from build123d import *

# Parameters (mm, degrees)
SKETCH001_W                   = 44
SKETCH001_H                   = 15
POCKET_DEPTH                  = 325.585135
PAD_DEPTH                     = 22.25
SKETCH003_W                   = 28
SKETCH003_H                   = 15
POCKET001_DEPTH               = 325.585135
SKETCH004_R                   = 1.5
POCKET002_DEPTH               = 45
SKETCH004_MIRRORED014_2_R     = 1.5
POCKET002_MIRRORED014_2_DEPTH = 45
SKETCH006_R                   = 1.2
POCKET004_DEPTH               = 325.585135
SKETCH006_MIRRORED016_2_R     = 1.2
POCKET004_MIRRORED016_2_DEPTH = 325.585135
SKETCH007_W                   = 3
SKETCH007_H                   = 11
PAD001_DEPTH                  = 11
SKETCH007_MIRRORED011_2_W     = 3
SKETCH007_MIRRORED011_2_H     = 11
PAD001_MIRRORED011_2_DEPTH    = 11
CYLINDER_R                    = 3.5
CYLINDER_DEPTH                = 33
CHAMFER_SIZE                  = 2


with BuildPart() as part:
    # Sketch → Revolution (revolve)
    with BuildSketch(Plane.XZ):
        Polygon((31, 0), (31, 14.5), (32, 16), (33.5, 14.5), (33.5, 2), (51.5, 2), (51.5, 14), (49.5, 16), (52.5, 16), (52.5, 18), (54, 18), (54, 0), align=None)
    revolve(axis=Axis((0, 0, 0), (0, 0, 1)))

    # Sketch001 → Pocket (cut, through all)
    with BuildSketch(Plane.XY):
        with Locations((0, 28.5)):
            Rectangle(SKETCH001_W, SKETCH001_H)
    pocket = extrude(amount=POCKET_DEPTH, mode=Mode.SUBTRACT)

    # Mirrored: Pocket across XZ
    add(pocket.mirror(Plane.XZ), mode=Mode.SUBTRACT)

    # Sketch002 → Pad (join, symmetric)
    with BuildSketch(Plane.YZ):
        Polygon((-40, 0), (-40, 6), (-32, 14), (-29, 14), (-29, 0), align=None)
    pad = extrude(amount=PAD_DEPTH, both=True)

    # Mirrored001: Pad across XZ
    add(pad.mirror(Plane.XZ))

    # Sketch003 → Pocket001 (cut, through all)
    with BuildSketch(Plane.XY):
        with Locations((0, 32.5)):
            Rectangle(SKETCH003_W, SKETCH003_H)
    pocket001 = extrude(amount=POCKET001_DEPTH, mode=Mode.SUBTRACT)

    # Mirrored002: Pocket001 across XZ
    add(pocket001.mirror(Plane.XZ), mode=Mode.SUBTRACT)

    # Sketch004 → Pocket002 (cut)
    with BuildSketch(Plane.XZ):
        with Locations((-18, 7)):
            Circle(SKETCH004_R)
    pocket002 = extrude(amount=-POCKET002_DEPTH, mode=Mode.SUBTRACT)

    # Sketch004 Mirrored014 2 → Pocket002 Mirrored014 2 (cut)
    with BuildSketch(Plane(origin=(0, 0, 0), x_dir=(-1, 0, 0), z_dir=(0, 1, 0))):
        with Locations((-18, 7)):
            Circle(SKETCH004_MIRRORED014_2_R)
    pocket002_mirrored014_2 = extrude(amount=POCKET002_MIRRORED014_2_DEPTH, mode=Mode.SUBTRACT)

    # Mirrored015: Pocket002, Pocket002 Mirrored014 2 across XZ
    add(pocket002.mirror(Plane.XZ), mode=Mode.SUBTRACT)
    add(pocket002_mirrored014_2.mirror(Plane.XZ), mode=Mode.SUBTRACT)

    # Sketch006 → Pocket004 (cut, through all)
    with BuildSketch(Plane.XY):
        with Locations((28.284271, 28.284271)):
            Circle(SKETCH006_R)
        with Locations((33.234019, 33.234019)):
            Circle(SKETCH006_R)
    pocket004 = extrude(amount=POCKET004_DEPTH, mode=Mode.SUBTRACT)

    # Sketch006 Mirrored016 2 → Pocket004 Mirrored016 2 (cut, through all)
    with BuildSketch(Plane(origin=(0, 0, 0), x_dir=(-1, 0, 0), z_dir=(0, 0, -1))):
        with Locations((28.284271, 28.284271)):
            Circle(SKETCH006_MIRRORED016_2_R)
        with Locations((33.234019, 33.234019)):
            Circle(SKETCH006_MIRRORED016_2_R)
    pocket004_mirrored016_2 = extrude(amount=-POCKET004_MIRRORED016_2_DEPTH, mode=Mode.SUBTRACT)

    # Mirrored017: Pocket004, Pocket004 Mirrored016 2 across XZ
    add(pocket004.mirror(Plane.XZ), mode=Mode.SUBTRACT)
    add(pocket004_mirrored016_2.mirror(Plane.XZ), mode=Mode.SUBTRACT)

    # Sketch007 → Pad001 (join)
    with BuildSketch(Plane.XY):
        with Locations((23.5, 27.5)):
            Rectangle(SKETCH007_W, SKETCH007_H)
    pad001 = extrude(amount=PAD001_DEPTH)

    # Sketch007 Mirrored011 2 → Pad001 Mirrored011 2 (add)
    with BuildSketch(Plane(origin=(0, 0, 0), x_dir=(-1, 0, 0), z_dir=(0, 0, -1))):
        with Locations((23.5, 27.5)):
            Rectangle(SKETCH007_MIRRORED011_2_W, SKETCH007_MIRRORED011_2_H)
    pad001_mirrored011_2 = extrude(amount=-PAD001_MIRRORED011_2_DEPTH)

    # Mirrored012: Pad001, Pad001 Mirrored011 2 across XZ
    add(pad001.mirror(Plane.XZ))
    add(pad001_mirrored011_2.mirror(Plane.XZ))

    # Cylinder → Cylinder (cut)
    with BuildSketch(Plane(origin=(33, 16, 6.5), x_dir=(1, 0, 0), z_dir=(0, -1, 0))):
        Circle(CYLINDER_R)
    cylinder = extrude(amount=CYLINDER_DEPTH, mode=Mode.SUBTRACT)

    # Mirrored013: Cylinder across YZ
    add(cylinder.mirror(Plane.YZ), mode=Mode.SUBTRACT)

    # Chamfer
    chamfer_edges = [part.edges().sort_by_distance(p)[0] for p in [
        (-54, 0, 0),
    ]]
    chamfer(chamfer_edges, length=CHAMFER_SIZE)


solid = part.part
Read the model definition and answer for the solid it produces. Units are mm, in the model's axes. A direction names the side the tool comes from. Round coordinates to 2 decimals unless told otherwise and drop trailing zeros. Loops run counter-clockwise (first coordinate to the right, second up) from the corner with the lowest first, then second, coordinate; pieces in that order, holes last. Notation, with made-up numbers: (27.25, 23) - (47.25, 23) arc R37 ccw to (47.25, 62) - close; hole circle Ø4 at (26, 10). An arc over 180 degrees is marked (long way). One line per question, with ' | ' between items. Start each with the question number.
Q1. Flat-ended cylindrical pins translate along their axes: pin 1 (1.5 mm diameter, centred on y = 17.5, z = 10.5, fed in from -X); pin 2 (2 mm diameter, centred on x = 7, z = 3.5, fed in from -Y); pin 3 (1 mm diameter, centred on x = 29.5, y = -26.5, fed in from +Z); pin 4 (4 mm diameter, centred on x = -6, y = -38.5, fed in from -Z). Find the tip coordinate at first contact, or state that the pin passes through.
Q2. Find the intervals of material crossed by L1, parallel to X at y = -32.5, z = 7; L2, parallel to Z at x = -18, y = -35; L3, parallel to Y at x = -21, z = 6.5, in increasing order.
Q3. Section A-A on x = 0 is taken. Give the vertices of the cut face in (y, z), plus the area to 3 significant figures.
Q4. Section B-B on y = 7.5 is taken. Count the separate pieces of the cut face and the enclosed holes in it, plus the area to 3 significant figures.
Q5. For faces 1 (the conical face through (24.053, -46.244, 0.125)), 2 (the flat face through (-25, -28, 6)), 3 (the flat face through (14, 33, 5)), determine the directions among +Z, -Z, +X, -X, +Y, -Y from which every point of the face is accessible in a straight line to the end or side of a thin tool.
Established:
1) pin 1: x = -51.34 | pin 2: y = -53.67 | pin 3: z = 2 | pin 4: z = 0
2) L1: -43.12 to -39.95, -25 to -19.5, -16.5 to -14, 14 to 16.5, 19.5 to 25, 39.95 to 43.12 | L2: 0 to 5.5, 8.5 to 11 | L3: -49.75 to -47.02, -39.5 to -29, 29 to 39.5, 47.02 to 49.75
3) outline: (-54, 2) - (-52, 0) - (-40, 0) - (-40, 2) - (-51.5, 2) - (-51.5, 14) - (-49.5, 16) - (-52.5, 16) - (-52.5, 18) - (-54, 18) - close; (40, 0) - (52, 0) - (54, 2) - (54, 18) - (52.5, 18) - (52.5, 16) - (49.5, 16) - (51.5, 14) - (51.5, 2) - (40, 2) - close | area: 132 mm²
4) separate pieces: 4 | enclosed holes: 0 | area: 208 mm²
5) face 1: -Z | face 2: +Z | face 3: +Z, -Z
